Geometry check sheet. Reference: the model listing, model coordinates, mm. Face numbers are marked on the shaded views. Round coordinates to 2 decimals unless told otherwise and drop trailing zeros. Order: outer loops, then holes, each group sorted by start corner. A loop starts at its lowest first (then second) coordinate and runs counter-clockwise, first axis right, second up.
(1) Draft check along X on the marked faces 1, 2 and 3. Enter one of: pulls with the +X half, pulls with the -X half, needs draft (parallel to the pull), parting line crosses it, or undercut.
(2) Cross-section at B-B on z = 0. Enter the section's corners in (x, y), and give its area (3 significant figures).
(3) Cross-section at A-A on x = 0. Enter the section's corners in (y, z).
(4) Cross-section at C-C on y = -2.5. Enter the section's corners in (x, z).
(5) Thickness scan on L1, parallel to X at y = -1.5, z = 18.5; L2, parallel to Z at x = 23, y = -1.75; L3, parallel to Z at x = 1.5, y = -2.25. Record the ranges inside material, lowest first.
(6) Cross-section at D-D on z = -10. Enter the section's corners in (x, y), and give its area (3 significant figures).
(7) Gauge pin test, flat ends, axial feed: P1, Ø2, axis at y = -1, z = -11, coming from the -X side; P2, Ø9, axis at x = 24.48, z = 14.13, coming from the -Y side; P3, Ø4, axis at x = -11, y = 0, coming from the -Z side; P4, Ø3, axis at y = -1.5, z = -8.5, coming from the -X side. Record the tip position at first contact, or that the pin passes through.
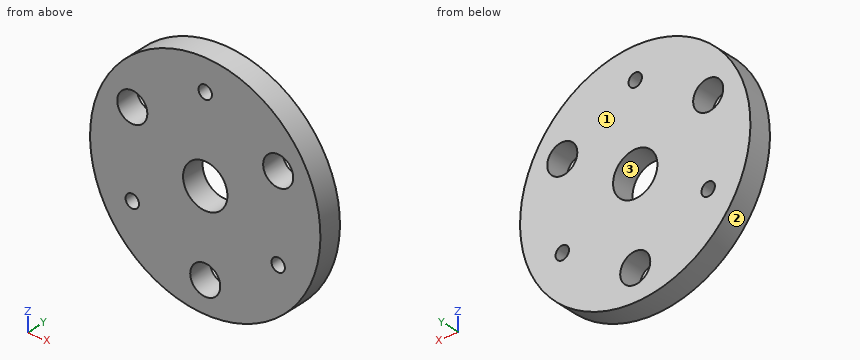
from build123d import *

# Parameters (mm, degrees)
SKETCH1_R               = 38.65245
SKETCH1_R_2             = 7.4422
BOSS_EXTRUDE1_DEPTH     = 3.8989
F_3_8_CLEARANCE_HOLE1_D = 10.0838
F_8_CLEARANCE_HOLE1_D   = 4.4958


with BuildPart() as part:
    # Sketch1 → Boss-Extrude1 (new, symmetric)
    with BuildSketch(Plane(origin=(0, 0, 0), x_dir=(1, 0, 0), z_dir=(0, 1, 0))):
        with Locations(Location((0, 0, 0), (0, 0, 270))):
            Circle(SKETCH1_R)
        with Locations(Location((0, 0, 0), (0, 0, 270))):
            Circle(SKETCH1_R_2, mode=Mode.SUBTRACT)
    extrude(amount=BOSS_EXTRUDE1_DEPTH, both=True)

    # 3/8 Clearance Hole1 (through all)
    with Locations(Plane(origin=(0, 3.8989, 0), x_dir=(1, 0, 0), z_dir=(0, 1, 0))):
        with Locations((0, 28.266203154), (24.47925, -14.133101577), (-24.47925, -14.133101577)):
            Hole(F_3_8_CLEARANCE_HOLE1_D / 2)

    # #8 Clearance Hole1 (through all)
    with Locations(Plane(origin=(0, 3.8989, 0), x_dir=(1, 0, 0), z_dir=(0, 1, 0))):
        with Locations((24.47925, 14.133101577), (0, -28.266203154), (-24.47925, 14.133101577)):
            Hole(F_8_CLEARANCE_HOLE1_D / 2)


solid = part.part
Found:
1. face 1: needs draft
1. face 2: parting line crosses it
1. face 3: undercut
2. outline: (-38.65, -3.9) - (-7.44, -3.9) - (-7.44, 3.9) - (-38.65, 3.9) - close; (7.44, -3.9) - (38.65, -3.9) - (38.65, 3.9) - (7.44, 3.9) - close
2. area: 487 mm2
3. outline: (-3.9, -38.65) - (3.9, -38.65) - (3.9, -33.31) - (-3.9, -33.31) - close; (-3.9, -23.22) - (3.9, -23.22) - (3.9, -7.44) - (-3.9, -7.44) - close; (-3.9, 7.44) - (3.9, 7.44) - (3.9, 26.02) - (-3.9, 26.02) - close; (-3.9, 30.51) - (3.9, 30.51) - (3.9, 38.65) - (-3.9, 38.65) - close
4. outline: circle Ø77.3 at (0, 0); hole circle Ø10.08 at (-24.48, 14.13); hole circle Ø4.5 at (-24.48, -14.13); hole circle Ø14.88 at (0, 0); hole circle Ø10.08 at (0, -28.27); hole circle Ø4.5 at (0, 28.27); hole circle Ø10.08 at (24.48, 14.13); hole circle Ø4.5 at (24.48, -14.13)
5. L1: x = -33.94 to -27, -21.96 to 21.96, 27 to 33.94
5. L2: z = -31.06 to -15.83, -12.44 to 9.31, 18.95 to 31.06
5. L3: z = -38.62 to -33.08, -23.45 to -7.29, 7.29 to 26.59, 29.94 to 38.62
6. outline: (-37.34, -3.9) - (37.34, -3.9) - (37.34, 3.9) - (-37.34, 3.9) - close
6. area: 582 mm2
7. P1: stops at x = -37.34
7. P2: passes through
7. P3: stops at z = -37.59
7. P4: stops at x = -38.01
